For this review, take the finished solid that the model builds, in its own axes (mm). A direction names the side the tool comes from. Coordinates: 2 decimals unless noted, no trailing zeros. Loops run counter-clockwise (first coordinate to the right, second up) from the corner with the lowest first, then second, coordinate; pieces in that order, holes last. Notation, with made-up numbers: M 67.25,52 L 95.25,52 A30 ccw 95.25,79 Z; hole C 10,-27.5 d4. An arc over 180 degrees is marked long. Put each result on its own line as item: value.
```python
from build123d import *

# Parameters (mm, degrees)
DODANIE_WYCI_GNI_CIE1_DEPTH      = 10
DODANIE_WYCI_GNI_CIE1_DEPTH_BACK = 10
SZKIC1_W                         = 70
SZKIC1_H                         = 20
SZKIC4_R                         = 5
DODANIE_WYCI_GNI_CIE2_DEPTH      = 40
SFAZOWANIE1_SIZE                 = 10
SFAZOWANIE1_SIZE_2               = 16.642794824
SZKIC5_W                         = 60
SZKIC5_H                         = 16
DODANIE_WYCI_GNI_CIE3_DEPTH      = 5
SZKIC6_W                         = 25
SZKIC6_H                         = 16
DODANIE_WYCI_GNI_CIE4_DEPTH      = 3


with BuildPart() as part:
    # Szkic1 → Dodanie-wyciągnięcie1 (new, two sides: drawn at the far end of the back side and taken through both)
    with BuildSketch(Plane.XY.offset(-DODANIE_WYCI_GNI_CIE1_DEPTH_BACK)):
        Rectangle(SZKIC1_W, SZKIC1_H)
    extrude(amount=DODANIE_WYCI_GNI_CIE1_DEPTH + DODANIE_WYCI_GNI_CIE1_DEPTH_BACK)

    # Wyciągnięcie po profilach1: read off the stored shape, not the designer's step
    # Wyciągnięcie po profilach1: loft between two sections, ruled curve by curve
    wyci_gni_cie_po_profilach1_from = [
        Edge.make_bspline([(-65, 1.414213562, -1.414213562), (-65, 1.580880229, -1.247546896), (-65, 1.730317192, -1.037358885), (-65, 1.94065032, -0.551350505), (-65, 2, -0.276142375), (-65, 2, 0.276142375), (-65, 1.94065032, 0.551350505), (-65, 1.730317192, 1.037358885), (-65, 1.580880229, 1.247546896), (-65, 1.414213562, 1.414213562)], [0, 0, 0, 0, 0.25, 0.25, 0.5, 0.5, 0.75, 0.75, 1, 1, 1, 1], 3),
        Edge.make_bspline([(-65, 1.414213562, 1.414213562), (-65, 1.247546896, 1.580880229), (-65, 1.037358885, 1.730317192), (-65, 0.551350505, 1.94065032), (-65, 0.276142375, 2), (-65, -0.276142375, 2), (-65, -0.551350505, 1.94065032), (-65, -1.037358885, 1.730317192), (-65, -1.247546896, 1.580880229), (-65, -1.414213562, 1.414213562)], [0, 0, 0, 0, 0.25, 0.25, 0.5, 0.5, 0.75, 0.75, 1, 1, 1, 1], 3),
        Edge.make_bspline([(-65, -1.414213562, -1.414213562), (-65, -1.247546896, -1.580880229), (-65, -1.037358885, -1.730317192), (-65, -0.551350505, -1.94065032), (-65, -0.276142375, -2), (-65, 0.276142375, -2), (-65, 0.551350505, -1.94065032), (-65, 1.037358885, -1.730317192), (-65, 1.247546896, -1.580880229), (-65, 1.414213562, -1.414213562)], [0, 0, 0, 0, 0.25, 0.25, 0.5, 0.5, 0.75, 0.75, 1, 1, 1, 1], 3),
        Edge.make_bspline([(-65, -1.414213562, 1.414213562), (-65, -1.580880229, 1.247546896), (-65, -1.730317192, 1.037358885), (-65, -1.94065032, 0.551350505), (-65, -2, 0.276142375), (-65, -2, -0.276142375), (-65, -1.94065032, -0.551350505), (-65, -1.730317192, -1.037358885), (-65, -1.580880229, -1.247546896), (-65, -1.414213562, -1.414213562)], [0, 0, 0, 0, 0.25, 0.25, 0.5, 0.5, 0.75, 0.75, 1, 1, 1, 1], 3),
    ]
    wyci_gni_cie_po_profilach1_to = [
        Edge.make_bspline([(-35, 10, -10), (-35, 10, -8.333333333), (-35, 10, -6.666666667), (-35, 10, -3.333333333), (-35, 10, -1.666666667), (-35, 10, 1.666666667), (-35, 10, 3.333333333), (-35, 10, 6.666666667), (-35, 10, 8.333333333), (-35, 10, 10)], [0, 0, 0, 0, 0.25, 0.25, 0.5, 0.5, 0.75, 0.75, 1, 1, 1, 1], 3),
        Edge.make_bspline([(-35, 10, 10), (-35, 8.333333333, 10), (-35, 6.666666667, 10), (-35, 3.333333333, 10), (-35, 1.666666667, 10), (-35, -1.666666667, 10), (-35, -3.333333333, 10), (-35, -6.666666667, 10), (-35, -8.333333333, 10), (-35, -10, 10)], [0, 0, 0, 0, 0.25, 0.25, 0.5, 0.5, 0.75, 0.75, 1, 1, 1, 1], 3),
        Edge.make_bspline([(-35, -10, -10), (-35, -8.333333333, -10), (-35, -6.666666667, -10), (-35, -3.333333333, -10), (-35, -1.666666667, -10), (-35, 1.666666667, -10), (-35, 3.333333333, -10), (-35, 6.666666667, -10), (-35, 8.333333333, -10), (-35, 10, -10)], [0, 0, 0, 0, 0.25, 0.25, 0.5, 0.5, 0.75, 0.75, 1, 1, 1, 1], 3),
        Edge.make_bspline([(-35, -10, 10), (-35, -10, 8.333333333), (-35, -10, 6.666666667), (-35, -10, 3.333333333), (-35, -10, 1.666666667), (-35, -10, -1.666666667), (-35, -10, -3.333333333), (-35, -10, -6.666666667), (-35, -10, -8.333333333), (-35, -10, -10)], [0, 0, 0, 0, 0.25, 0.25, 0.5, 0.5, 0.75, 0.75, 1, 1, 1, 1], 3),
    ]
    wyci_gni_cie_po_profilach1 = Solid(Shell([*[Face.make_surface_from_curves(wyci_gni_cie_po_profilach1_from[k], wyci_gni_cie_po_profilach1_to[k]) for k in range(4)], Face(Wire(wyci_gni_cie_po_profilach1_from)), Face(Wire(wyci_gni_cie_po_profilach1_to))]))
    add(wyci_gni_cie_po_profilach1)

    # Szkic4 → Dodanie-wyciągnięcie2 (add)
    with BuildSketch(Plane(origin=(35, 0, 0), x_dir=(0, 0, -1), z_dir=(1, 0, 0))):
        Circle(SZKIC4_R)
    extrude(amount=DODANIE_WYCI_GNI_CIE2_DEPTH)

    # Sfazowanie1
    # the kernel refuses this chamfer: 16.642794824, 10 mm, written as the material it adds along each edge
    with BuildSketch(Plane(origin=(35, 0, 0), x_dir=(0, 0, -1), z_dir=(0, -1, 0))) as sfazowanie1_piece_1_section:
        Polygon((5 + SFAZOWANIE1_SIZE, 0), (5, SFAZOWANIE1_SIZE_2), (5, 0), align=None)
    sfazowanie1_piece_1 = revolve(axis=Axis((35, 0, 0), (1, 0, 0)), mode=Mode.PRIVATE)
    sfazowanie1_piece_1 = split(sfazowanie1_piece_1, bisect_by=Plane(origin=(35, 10, 0), z_dir=(0, -1, 0)), keep=Keep.TOP, mode=Mode.PRIVATE)
    sfazowanie1_piece_1 = split(sfazowanie1_piece_1, bisect_by=Plane(origin=(35, 0, 10), z_dir=(0, 0, -1)), keep=Keep.TOP, mode=Mode.PRIVATE)
    sfazowanie1_piece_1 = split(sfazowanie1_piece_1, bisect_by=Plane(origin=(35, 0, -10), z_dir=(0, 0, 1)), keep=Keep.TOP, mode=Mode.PRIVATE)
    sfazowanie1_piece_1 = split(sfazowanie1_piece_1, bisect_by=Plane(origin=(35, -10, 0), z_dir=(0, 1, 0)), keep=Keep.TOP, mode=Mode.PRIVATE)
    add(sfazowanie1_piece_1)

    # Szkic5 → Dodanie-wyciągnięcie3 (add)
    with BuildSketch(Plane(origin=(0, 10, 0), x_dir=(1, 0, 0), z_dir=(0, 1, 0))):
        Rectangle(SZKIC5_W, SZKIC5_H)
    extrude(amount=DODANIE_WYCI_GNI_CIE3_DEPTH)

    # Szkic6 → Dodanie-wyciągnięcie4 (add)
    with BuildSketch(Plane(origin=(0, 15, 0), x_dir=(1, 0, 0), z_dir=(0, 1, 0))):
        with Locations((-17.5, 0)):
            Rectangle(SZKIC6_W, SZKIC6_H)
    extrude(amount=DODANIE_WYCI_GNI_CIE4_DEPTH)


solid = part.part
```
(1) Wall thickness on line 1 along X through (y, z) = (15.25, 5); line 2 along Y through (x, z) = (32, 6.5); line 3 along Y through (x, z) = (3, -3.75): over which ranges is each line inside the solid? List them lowest first. Write a range as [from, to].
Determined:
line 1: x = [-30, -5]
line 2: y = [-10, 10]
line 3: y = [-10, 15]
(2) Add section A-A (x = 32). Write out the cut boundary in (y, z), plus the area to 3 significant figures.
Determined:
outline: M -10,-10 L 10,-10 L 10,10 L -10,10 Z
area: 400 mm^2
(3) For pin 1 (3 mm diameter, centred on y = 8, z = -4.5, fed in from +X); pin 2 (9 mm diameter, centred on x = -14, y = 15, fed in from +Z); pin 3 (3 mm diameter, centred on x = 19.5, z = 6, fed in from +Y), all flat-tipped, find the tip position at first contact; note any pin that passes through.
Determined:
pin 1: stops at x = 47.18
pin 2: stops at z = 8
pin 3: stops at y = 15
(4) Tool access review of faces 1 (the flat face through (-5, 16, 0)), 2 (the cylindrical face through (63.16, -4.88, 1.08)), 3 (the flat face through (-30, 14, 0)), 4 (the flat face through (0, 13, 8)): name each direction out of +Z, -Z, +X, -X, +Y, -Y from which nothing blocks a thin tool from reaching the whole face with its end or side.
Determined:
face 1: +Z, -Z, +X, +Y
face 2: +X
face 3: +Z, -Z, -X, +Y
face 4: +Z, +X, -X, +Y
